Source: three-view drawing plus pictorial views. Frame: mm from the lowest corner of the part. Round coordinates to 2 decimals unless told otherwise and drop trailing zeros. Loops run counter-clockwise (first coordinate to the right, second up) from the corner with the lowest first, then second, coordinate; pieces in that order, holes last. Notation, with made-up numbers: M 81.25,46 L 139.25,46 A8 cw 139.25,58 Z; hole C 44.25,11 d11. An arc over 180 degrees is marked long. Answer as a JSON object with one key per item and string values.
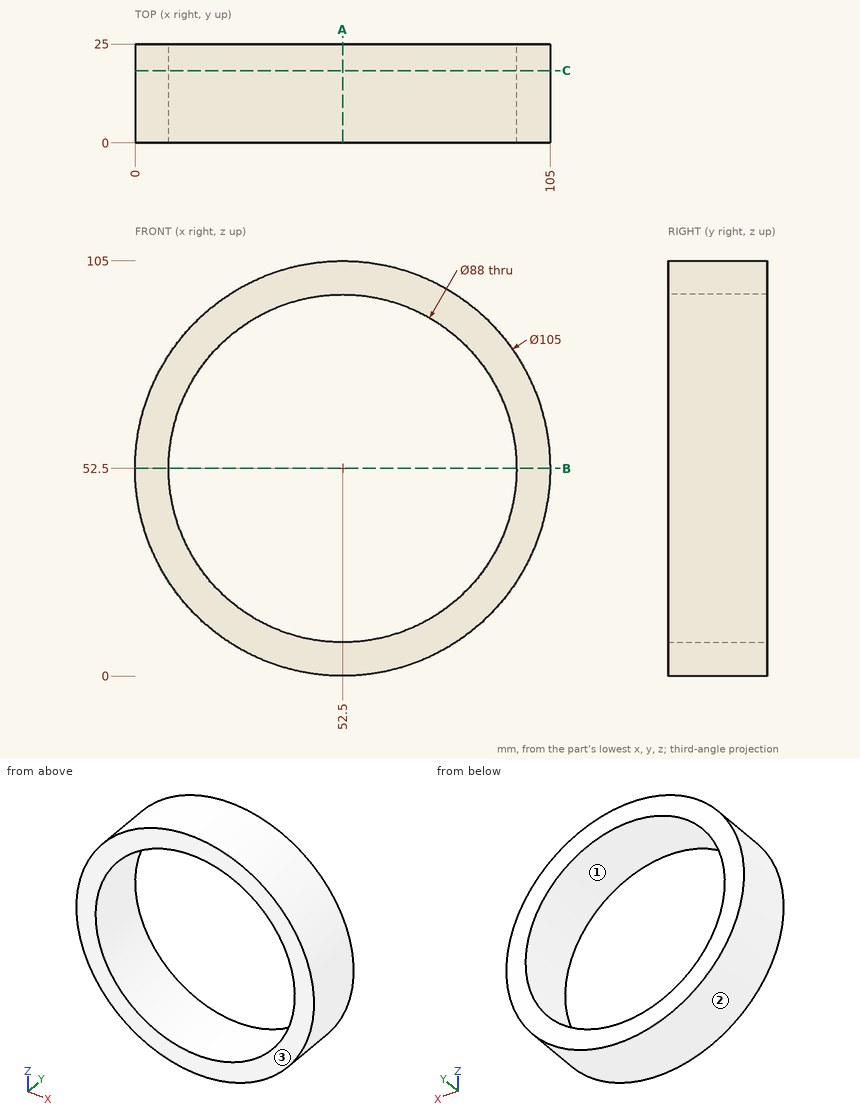
1) First-contact query: pin 1 (2 mm diameter, centred on y = 3.5, z = 68, fed in from -X); pin 2 (3 mm diameter, centred on y = 10.5, z = 17.5, fed in from -X); pin 3 (6 mm diameter, centred on y = 21, z = 47, fed in from +X). Flat tips, straight axial feed; report the tip coordinate or a pass-through.
Geometry results:
{"pin 1": "x = 2.04", "pin 2": "x = 12.08", "pin 3": "x = 104.94"}
2) Pull-direction query (X, two-part tool) for the marked faces 1, 2 and 3; classes: +X half, -X half, draft (parallel to the pull), parting line (faces both ways), or undercut.
Geometry results:
{"face 1": "undercut", "face 2": "parting line", "face 3": "draft"}
3) Cut plane A-A on x = 52.5. Return the cut outline in (y, z), and give its area (3 significant figures).
Geometry results:
{"outline": "M 0,0 L 25,0 L 25,8.5 L 0,8.5 Z; M 0,96.5 L 25,96.5 L 25,105 L 0,105 Z", "area": "425 mm2"}
4) Cut plane B-B on z = 52.5. Return the cut outline in (x, y), and give its area (3 significant figures).
Geometry results:
{"outline": "M 0,0 L 8.5,0 L 8.5,25 L 0,25 Z; M 96.5,0 L 105,0 L 105,25 L 96.5,25 Z", "area": "425 mm2"}
5) Line query: probe 1 along X at (y, z) = (13, 51); probe 2 along X at (y, z) = (14.75, 72); probe 3 along Z at (x, y) = (18, 19.75). Output: solid intervals per line, ascending.
Geometry results:
{"probe 1": "0.02 to 8.53, 96.47 to 104.98", "probe 2": "3.76 to 13.06, 91.94 to 101.24", "probe 3": "12.93 to 25.19, 79.81 to 92.07"}
6) Cut plane C-C on y = 18.25. Return the cut outline in (x, z).
Geometry results:
{"outline": "C 52.5,52.5 d105; hole C 52.5,52.5 d88"}
